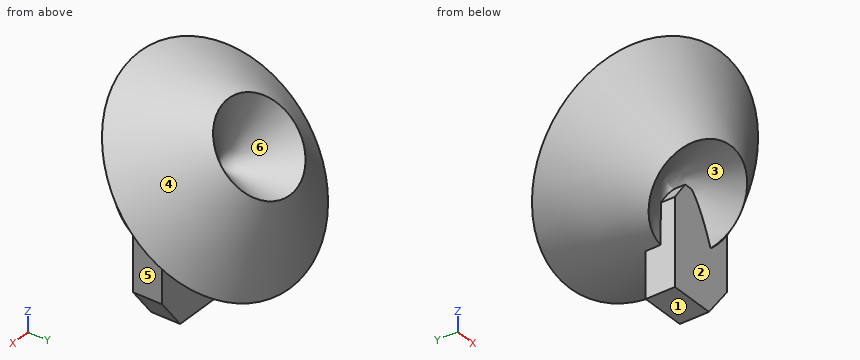
```python
from build123d import *

# Parameters (mm, degrees)
F1_DEPTH = 25.4


with BuildPart() as f1:
    # F0 (on Front) → F1 (new body)
    with BuildSketch(Plane.XZ):
        Polygon((54.5106306672, 36.1877307296), (6.2173682239, 36.1877307296), (-5.6495610625, 19.6164111685), (-5.6495610625, -55.4267726839), (33.7284366412, -55.4267726839), (54.5106306672, -28.1047300409), align=None)
    extrude(amount=F1_DEPTH)

    # F2 (on Right) → F3 (revolve)
    with BuildSketch(Plane.YZ):
        Polygon((70.0851008296, 61.8397891521), (10.0763916288, 61.8397891521), (-12.6733398065, 41.4988532085), (-12.6733398065, -15.7271567732), (70.0851008296, -15.7271567732), align=None)
    revolve(axis=Axis((0, -4.0846643969, 49.1781393066), (0, -0.7454706515, -0.6665384518)))


solid = f1.part
```
Geometry: final body of the model. Coordinates: model frame, mm. Face numbers are marked on the shaded views. A direction names the side the tool comes from. Coordinates: 2 decimals unless noted, no trailing zeros. Order: outer loops, then holes, each group sorted by start corner. A loop starts at its lowest first (then second) coordinate and runs counter-clockwise, first axis right, second up. Notation, with made-up numbers: (38.25, 86.5) - (62.25, 86.5) arc R16 ccw to (62.25, 107.5) - close; hole circle Ø6 at (51, -10.5). An arc over 180 degrees is marked (long way). Return JSON: item names as keys, results as strings. Group by question number.
1. Set-up query: the marked faces 1 and 2. Return all of +Z, -Z, +X, -X, +Y, -Y with unobstructed straight access to the full face (end or side cutting, diameter ignored); none if empty.
2. Cut plane A-A (z = -31.5). Output: boundary loops of the cut face in (x, y), plus the area to 3 significant figures.
3. Material intervals for line 1 along X through (y, z) = (54.5, 72.5); line 2 along X through (y, z) = (47, 73.5); line 3 along X through (y, z) = (-36, 115.5), sorted ascending. Write a range as [from, to].
4. Pull-direction query (X, two-part tool) for the marked faces 3, 4, 5 and 6; classes: pulls with the +X half, pulls with the -X half, needs draft (parallel to the pull), parting line crosses it, or undercut.
5. Pin query (flat end, axial travel): pin 1 (10 mm diameter, centred on x = -9, z = 109.5, fed in from +Y); pin 2 (2 mm diameter, centred on x = 10, y = 46.5, fed in from +Z); pin 3 (12 mm diameter, centred on x = 48.5, z = 87.5, fed in from -Y). Return the tip coordinate at first contact, or that it passes through.
Resolved:
{
 "1": {"face 1": "-Z, +X, -X, +Y, -Y", "face 2": "-Z, -Y"},
 "2": {"outline": "(-5.65, -25.4) - (51.93, -25.4) - (51.93, 0) - (-5.65, 0) - close", "area": "1,460 mm²"},
 "3": {"line 1": "x = [-39.49, -28.71], [28.71, 39.49]", "line 2": "x = [-47.98, -27.25], [27.25, 47.98]", "line 3": "x = [-53.12, 53.12]"},
 "4": {"face 3": "undercut", "face 4": "parting line crosses it", "face 5": "pulls with the +X half", "face 6": "undercut"},
 "5": {"pin 1": "stops at y = 17.75", "pin 2": "stops at z = 63.71", "pin 3": "stops at y = -55.32"}
}
